from build123d import *

# Parameters (mm, degrees)
SKETCH16_R         = 52.5
SKETCH16_R_2       = 50.8
CUT_EXTRUDE1_DEPTH = 11.43


with BuildPart() as part:
    # Sketch1 → Bearing Shaft/Flange Support (revolve)
    with BuildSketch(Plane(origin=(0, 0, 0), x_dir=(0, 0, -1), z_dir=(1, 0, 0)), mode=Mode.PRIVATE) as bearing_shaft_flange_support_sk:
        Polygon((0, 0), (-27.254672075, 0), (-25.0825, -12.319), (-25.0825, -17.0815), (-15.875, -17.0815), (-15.875, -69.56298), (-14.2875, -71.15048), (0, -71.15048), align=None)
    revolve(bearing_shaft_flange_support_sk.sketch.rotate(Axis((0, 0, 0), (0, 1, 0)), 180), axis=Axis((0, 0, 0), (0, 1, 0)))

    # Sketch2 → Drive Pin Support (revolve)
    with BuildSketch(Plane(origin=(0, 0, 0), x_dir=(0, 0, -1), z_dir=(1, 0, 0)), mode=Mode.PRIVATE) as drive_pin_support_sk:
        Polygon((0, 0), (-52.5, 0), (-52.5, 11.43), (-27.4096, 11.43), (-27.4096, 18.43), (-22.225, 18.43), (-22.225, 27.305), (-23.61946, 27.305), (-23.61946, 68.2625), (-22.03196, 69.85), (0, 69.85), align=None)
    revolve(drive_pin_support_sk.sketch.rotate(Axis((0, 0, 0), (0, 1, 0)), 180), axis=Axis((0, 0, 0), (0, 1, 0)))

    # Sketch16 → Cut-Extrude1 (cut)
    with BuildSketch(Plane(origin=(0, 11.43, 0), x_dir=(1, 0, 0), z_dir=(0, 1, 0))):
        Circle(SKETCH16_R)
        with Locations(Location((0, 0, 0), (0, 0, 270))):
            Circle(SKETCH16_R_2, mode=Mode.SUBTRACT)
    extrude(amount=-CUT_EXTRUDE1_DEPTH, mode=Mode.SUBTRACT)


solid = part.part
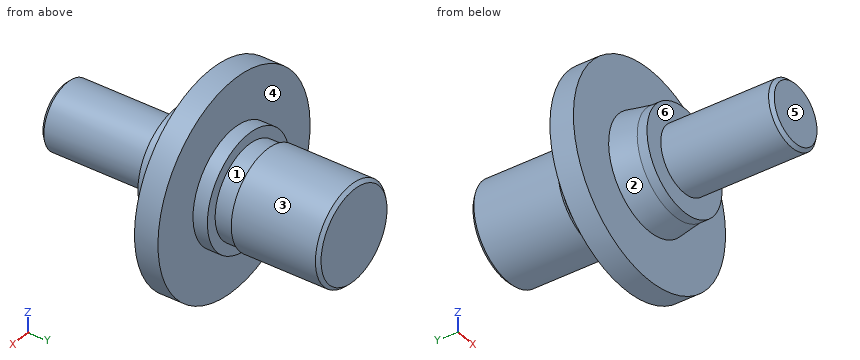
Work out the finished part from the listing and answer in its coordinate system (mm). Face numbers are marked on the shaded views. A direction names the side the tool comes from. Give positions to 0.01 mm unless a question says otherwise; leave off trailing zeros. Loops run counter-clockwise (first coordinate to the right, second up) from the corner with the lowest first, then second, coordinate; pieces in that order, holes last. Notation, with made-up numbers: M 68.25,-3.5 L 83.25,-3.5 A37 cw 83.25,34.5 Z; hole C -12,66.5 d11. An arc over 180 degrees is marked long. Use CSV: the item, a comma, the result in double quotes.
1) Find section C-C on y = -40. Write down the section's boundary in (x, z) (3 decimals), plus the area to 3 significant figures.
Answer:
outline,"C 0,0 d31.75"
area,"792 mm^2"
2) Given P1, Ø1.5, axis at x = 7, y = -39.5, coming from the -Z side; P2, Ø5, axis at x = 19, z = -32.5, coming from the +Y side; P3, Ø1.5, axis at x = 10.5, y = -10, coming from the -Z side; P4, Ø3, axis at y = -2.5, z = -38, coming from the -X side, each flat-ended and moving along its own axis, determine where each tip first touches the part or whether it passes through.
Answer:
P1,"z = -14.59"
P2,"y = 11.43"
P3,"z = -23.58"
P4,"through"
3) Which of the six approach directions +Z, -Z, +X, -X, +Y, -Y give full straight-line access (tool end or side, diameter ignored) to the marked faces 4, 5 and 6?
Answer:
face 4,"+Y"
face 5,"+Z, -Z, +X, -X, -Y"
face 6,"-Y"
4) Find section D-D on x = -39. Write down the section's boundary in (y, z).
Answer:
outline,"M 0,-32.55 L 11.43,-32.55 L 11.43,32.55 L 0,32.55 Z"
5) Determine the mould class of the marked faces 1, 2 and 3 for opening direction Y: released by +Y, released by -Y, zero draft, split by the parting line, or undercut.
Answer:
face 1,"undercut"
face 2,"released by -Y"
face 3,"zero draft"
6) Consider L1, parallel to Y at x = -22, z = 29; L2, parallel to X at y = 61, z = 0; L3, parallel to X at y = -42, z = 0 (3 decimals). Determine where each line is inside the solid, lowest interval first.
Answer:
L1,"0 to 11.43"
L2,"-23.62 to 23.62"
L3,"-15.875 to 15.875"
